Build history of the part. All positions in model axes, mm. Round coordinates to 2 decimals unless told otherwise and drop trailing zeros. Order: outer loops, then holes, each group sorted by start corner. A loop starts at its lowest first (then second) coordinate and runs counter-clockwise, first axis right, second up. Notation, with made-up numbers: (31.5, 65) -> (48.5, 65) arc R13 ccw to (48.5, 70) -> close; hole circle Ø6 at (21.25, 14). An arc over 180 degrees is marked (long way). Use a Markdown table: item, result. Add a question column.
Item 1: Slice it at A-A, the plane z = 0. Give the cut face in (x, y), plus the area to 3 significant figures.
Item 2: Slice it at B-B, the plane x = 0. Give the cut face in (y, z).
Item 3: Probe L1, parallel to X at y = 20, z = 1.75; L2, parallel to Y at x = 0, z = 0.5; L3, parallel to Y at x = -2.5, z = -3.5. List the from-to ranges inside material, lowest first.
Item 4: Pin check, flat tips, straight feed: pin 1 (1.5 mm diameter, centred on x = 0.5, y = 22.5, fed in from -Z); pin 2 (6 mm diameter, centred on y = 24.5, z = -1.5, fed in from +X); pin 3 (6 mm diameter, centred on y = 11, z = 3.5, fed in from -X); pin 4 (5 mm diameter, centred on x = 0.5, z = -3, fed in from +Y). Stop position of each tip, or through.
Item 5: Slice it at D-D, the plane y = 13.5. Give the cut face in (x, z).
Item 6: Slice it at C-C, the plane y = 21.75. Give the cut face in (x, z).
Autodesk Inventor part; units mm, degrees
ref_plane "YZ Plane" through (0, 0, 0) normal (1, 0, 0) x (0, 1, 0)
ref_plane "XZ Plane" through (0, 0, 0) normal (0, 1, 0) x (-1, 0, 0)
ref_plane "XY Plane" through (0, 0, 0) normal (0, 0, 1) x (1, 0, 0)
sketch "Sketch1" plane through (0, 0, 0) normal (0, 1, 0) x (-1, 0, 0)
  circle A0 centre (0, 0) radius 4.65
  dimension "d0" = 9.3
extrude "Extrusion1" add sketch "Sketch1" along normal blind 15.45
sketch "Sketch2" plane through (0, 0, 0) normal (1, 0, 0) x (0, 1, 0)
  line L0 (15.45, -4.65) -> (15.45, 4.65)
  line L1 (0, -4.65) -> (0, 4.65)
  line L2 (0, -4.65) -> (15.45, -4.65)
  line L3 (0, 4.65) -> (15.45, 4.65)
  line L4 (0, -4.65) -> (1, -4.65)
  arc A0 (2.5, -4.65) -> (1, -4.65) centre (1.75, -4.65) ccw
  line L5 (2.5, -4.65) -> (1, -4.65)
  line L6 (-3.09, 0) -> (18.54, 0)
  point P0 (0, 0)
  dimension "d3" = 1
  dimension "d4" = 1.5
  dimension "d5" = 0.75
revolve "Revolution1" cut sketch "Sketch2" angle 360 about axis through (0, -10, 0) along (0, 1, 0) contours L2 A0
sketch "Sketch3" plane through (0, 15.45, 0) normal (0, 1, 0) x (1, 0, 0)
  circle A0 centre (0, 0) radius 4.65
  line L0 (0, 0) -> (0, 4.65)
  line L1 (0, 5.55) -> (0.5, 5.55)
  line L2 (0, 5.55) -> (-0.5, 5.55)
  line L3 (-0.5, 5.55) -> (-0.5, 4.623)
  line L4 (0.5, 5.55) -> (0.5, 4.623)
  circle A1 centre (0, 0) radius 4.65
  dimension "d7" = 0.9
  dimension "d8" = 0.5
  dimension "d9" = 0.5
extrude "Extrusion2" add sketch "Sketch3" against normal blind 0.25 contours A0 L3 L2 L1 L4
sketch "Sketch5" plane through (0, 15.45, 0) normal (0, 1, 0) x (1, 0, 0)
  arc A0 (-0.5, 4.623) -> (0.5, 4.623) centre (0, 0) ccw
  line L0 (0.5, 4.623) -> (0.5, 5.55)
  line L1 (0.5, 5.55) -> (-0.5, 5.55)
  line L2 (-0.5, 5.55) -> (-0.5, 4.623)
  line L3 (0, 0) -> (4.65, 0) construction
  line L4 (0, 0) -> (1.7961, 1.7961) construction
  circle A1 centre (1.781, 1.781) radius 0.1
  line L5 (1.781, 1.781) -> (1.781, 0) construction
  circle A2 centre (1.781, -1.781) radius 0.1
  line L6 (0, 0) -> (0, 5.55) construction
  circle A3 centre (-1.781, 1.781) radius 0.1
  circle A4 centre (-1.781, -1.781) radius 0.1
  circle A5 centre (-1.781, 1.781) radius 0.15
  dimension "d14" = 2.54
  dimension "d15" = 45
  dimension "d16" = 0.2
  dimension "d17" = 1.781
  dimension "d20" = 3.562
  dimension "d27" = 0.05
extrude "Extrusion3" add sketch "Sketch5" along normal blind 13.5 contours A1 | A2 | A3 | A4
extrude "Extrusion4" add sketch "Sketch5" along normal blind 0.25 contours A5
chamfer "Chamfer1" distance 0.05 angle 45 1 edges at (-1.931, 15.7, -1.781)
properties part number "IR Sensor"
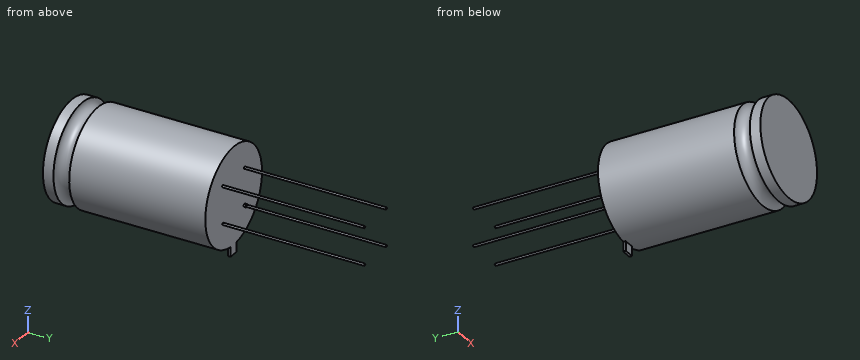
Check sheet entries:
| question | item | result |
|---|---|---|
| 1 | outline | (-4.65, 0) -> (4.65, 0) -> (4.65, 1) arc R0.75 cw to (4.65, 2.5) -> (4.65, 15.45) -> (-4.65, 15.45) -> (-4.65, 2.5) arc R0.75 cw to (-4.65, 1) -> close |
| 1 | area | 142 mm2 |
| 2 | outline | (0, -4.65) -> (1, -4.65) arc R0.75 cw to (2.5, -4.65) -> (15.2, -4.65) -> (15.2, -5.55) -> (15.45, -5.55) -> (15.45, 4.65) -> (2.5, 4.65) arc R0.75 cw to (1, 4.65) -> (0, 4.65) -> close |
| 3 | L1 | -1.88 to -1.69, 1.69 to 1.88 |
| 3 | L2 | 0 to 15.45 |
| 3 | L3 | 0 to 1.09, 2.41 to 15.45 |
| 4 | pin 1 | through |
| 4 | pin 2 | x = 1.88 |
| 4 | pin 3 | x = -4.62 |
| 4 | pin 4 | y = 28.95 |
| 5 | outline | circle Ø9.3 at (0, 0) |
| 6 | outline | circle Ø0.2 at (-1.78, -1.78); circle Ø0.2 at (-1.78, 1.78); circle Ø0.2 at (1.78, -1.78); circle Ø0.2 at (1.78, 1.78) |
